Answer from the drawing. Dimensions are ordinates in mm from the lowest x, y and z of the part. A direction names the side the tool comes from. Give positions to 0.01 mm unless a question says otherwise; leave off trailing zeros. Order: outer loops, then holes, each group sorted by start corner. A loop starts at its lowest first (then second) coordinate and runs counter-clockwise, first axis right, second up. Notation, with made-up numbers: (-20.5, 4.5) - (15.5, 4.5) arc R27 cw to (15.5, 41.5) - close; hole circle Ø7 at (26, 37). An arc over 180 degrees is marked (long way). Write each question's results on one line, items separated by ' | '.
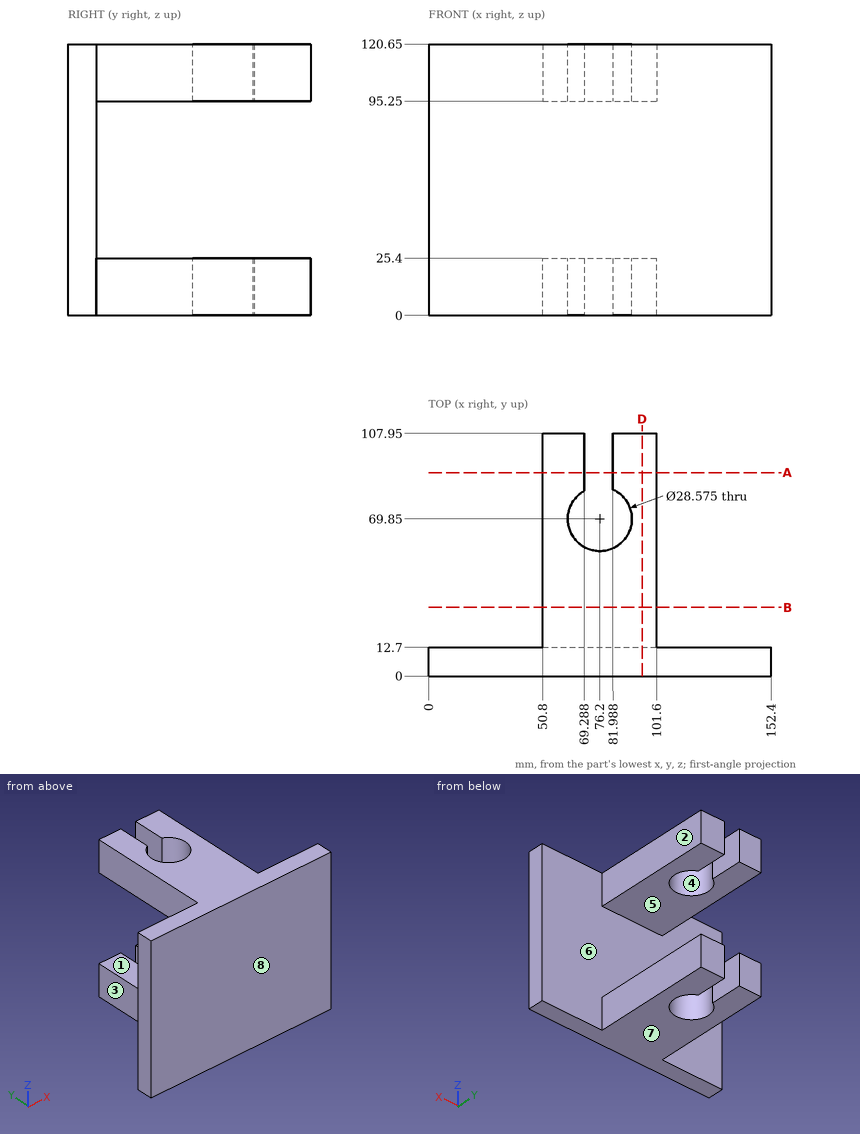
1. Straight lines are drawn through the part: line 1 (X direction, y = 69.85, z = 14); line 2 (Z direction, x = 61, y = 42); line 3 (Y direction, x = 45.5, z = 58). For each, find the intervals that lie inside material, in ascending order. Write a range as [from, to].
Answer list:
line 1: [50.8, 61.91], [90.49, 101.6] | line 2: [0, 25.4], [95.25, 120.65] | line 3: [0, 12.7]
2. A cutting plane is placed at D-D, the plane x = 95. Write down the section's boundary in (y, z).
Answer list:
outline: (0, 0) - (107.95, 0) - (107.95, 25.4) - (12.7, 25.4) - (12.7, 95.25) - (107.95, 95.25) - (107.95, 120.65) - (0, 120.65) - close
3. A cutting plane is placed at A-A, the plane y = 90.5. Write down the section's boundary in (x, z).
Answer list:
outline: (50.8, 0) - (69.29, 0) - (69.29, 25.4) - (50.8, 25.4) - close; (50.8, 95.25) - (69.29, 95.25) - (69.29, 120.65) - (50.8, 120.65) - close; (81.99, 0) - (101.6, 0) - (101.6, 25.4) - (81.99, 25.4) - close; (81.99, 95.25) - (101.6, 95.25) - (101.6, 120.65) - (81.99, 120.65) - close
4. A tool of negligible diameter and unlimited length cuts with its end or side. For the marked faces 1, 2, 3 and 4, from which of +Z, -Z, +X, -X, +Y, -Y can it reach the whole face along a straight path? Write none if from no direction.
Answer list:
face 1: +X, -X, +Y | face 2: +Z, -Z, +X, +Y | face 3: +Z, -Z, -X, +Y | face 4: +Z, -Z
5. A cutting plane is placed at B-B, the plane y = 30.5. Write down the section's boundary in (x, z), then the cut area to 3 significant figures.
Answer list:
outline: (50.8, 0) - (101.6, 0) - (101.6, 25.4) - (50.8, 25.4) - close; (50.8, 95.25) - (101.6, 95.25) - (101.6, 120.65) - (50.8, 120.65) - close | area: 2,580 mm^2
6. Determine the mould class of the marked faces 5, 6, 7 and 8 for opening direction Z: +Z half, -Z half, draft (parallel to the pull), parting line (faces both ways), or undercut.
Answer list:
face 5: undercut | face 6: undercut | face 7: -Z half | face 8: draft
7. Given P1, Ø7.5, axis at y = 92.5, z = 105.5, coming from the +X side; P2, Ø23, axis at x = 76.2, y = 69.85, coming from the +Z side; P3, Ø12.5, axis at y = 79, z = 10, coming from the -X side; P4, Ø1, axis at x = 76.5, z = 65, coming from the -Y side, each flat-ended and moving along its own axis, determine where each tip first touches the part or whether it passes through.
Answer list:
P1: x = 101.6 | P2: through | P3: x = 50.8 | P4: y = 0
